Answer from the drawing. Dimensions are ordinates in mm from the lowest x, y and z of the part. A direction names the side the tool comes from. Give positions to 0.01 mm unless a question says otherwise; leave off trailing zeros. Order: outer loops, then holes, each group sorted by start corner. A loop starts at its lowest first (then second) coordinate and runs counter-clockwise, first axis right, second up. Notation, with made-up numbers: (50.25, -28) - (60.25, -28) arc R23 cw to (60.25, -20) - close; hole circle Ø2 at (55, -27.5). An arc over 180 degrees is marked (long way). Answer in a Markdown table with one row per item. Add a question column.
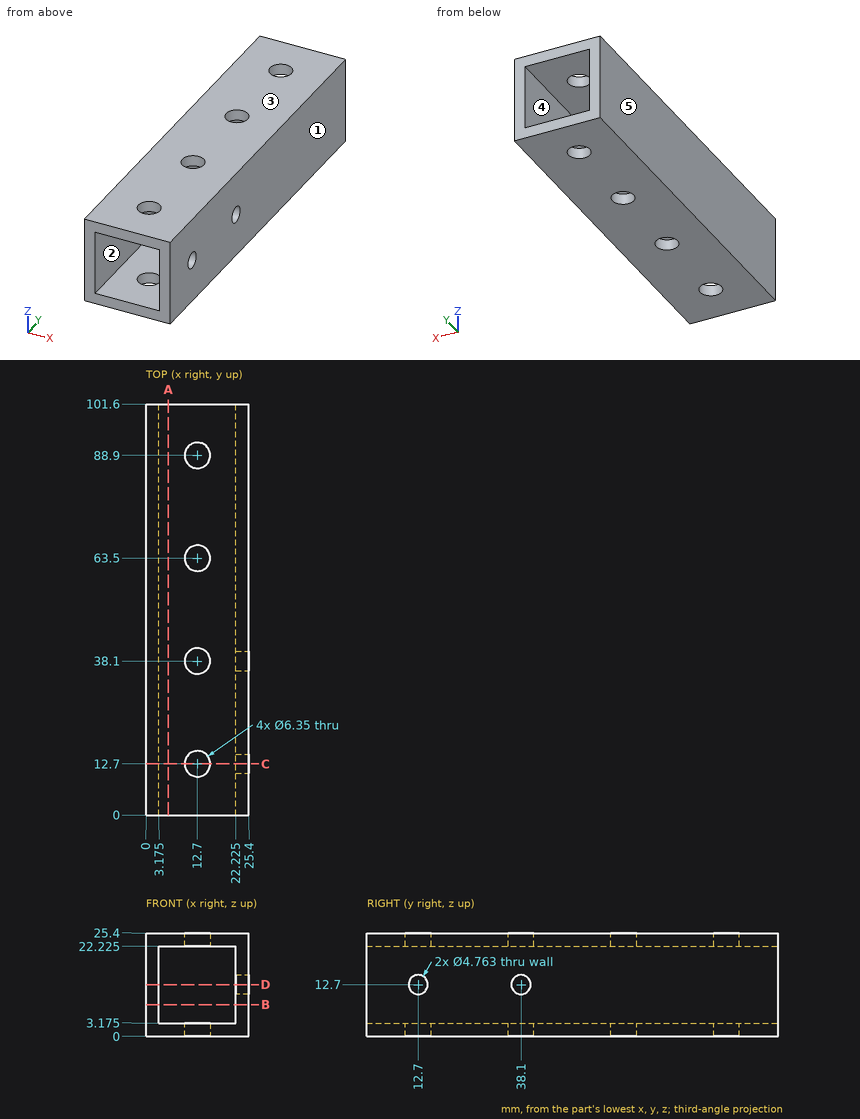
(1) Each of these flat-tipped pins is pushed along its axis until it touches: P1, Ø2, axis at x = 14.5, y = 36.5, coming from the -Z side; P2, Ø4, axis at y = 12.7, z = 12.7, coming from the +X side (1 decimal). Where does it stop, or does it pass through?
(2) Find section C-C, the plane y = 12.7. Write down the section's boundary in (x, z) (1 decimal), plus the area to 3 significant figures.
(3) Find section A-A, the plane x = 5.5. Write down the section's boundary in (y, z) (1 decimal).
(4) Find section B-B, the plane z = 7.75. Write down the section's boundary in (x, y) (1 decimal).
(5) Straight lines are drawn through the part: line 1 (Y direction, x = 12.7, z = 23.2) (1 decimal); line 2 (X direction, y = 37, z = 20.25) (1 decimal). For each, find the intervals that lie inside material, in ascending order.
(6) The mould has two halves that part along X. Classify the marked faces 1, 2 and 3: +X half, -X half, draft (parallel to the pull), parting line (faces both ways), or undercut.
(7) Find section D-D, the plane z = 12.7. Write down the section's boundary in (x, y) (1 decimal).
(8) For the marked faces 4 and 5, determine the directions among +Z, -Z, +X, -X, +Y, -Y from which every point of the face is accessible in a straight line to the end or side of a thin tool.
Answer key:
| question | item | result |
|---|---|---|
| 1 | P1 | z = 0 |
| 1 | P2 | x = 3.2 |
| 2 | outline | (0, 0) - (9.5, 0) - (9.5, 3.2) - (3.2, 3.2) - (3.2, 22.2) - (9.5, 22.2) - (9.5, 25.4) - (0, 25.4) - close; (15.9, 0) - (25.4, 0) - (25.4, 10.3) - (22.2, 10.3) - (22.2, 3.2) - (15.9, 3.2) - close; (15.9, 22.2) - (22.2, 22.2) - (22.2, 15.1) - (25.4, 15.1) - (25.4, 25.4) - (15.9, 25.4) - close |
| 2 | area | 227 mm² |
| 3 | outline | (0, 0) - (101.6, 0) - (101.6, 3.2) - (0, 3.2) - close; (0, 22.2) - (101.6, 22.2) - (101.6, 25.4) - (0, 25.4) - close |
| 4 | outline | (0, 0) - (3.2, 0) - (3.2, 101.6) - (0, 101.6) - close; (22.2, 0) - (25.4, 0) - (25.4, 101.6) - (22.2, 101.6) - close |
| 5 | line 1 | 0 to 9.5, 15.9 to 34.9, 41.3 to 60.3, 66.7 to 85.7, 92.1 to 101.6 |
| 5 | line 2 | 0 to 3.2, 22.2 to 25.4 |
| 6 | face 1 | +X half |
| 6 | face 2 | undercut |
| 6 | face 3 | draft |
| 7 | outline | (0, 0) - (3.2, 0) - (3.2, 101.6) - (0, 101.6) - close; (22.2, 0) - (25.4, 0) - (25.4, 10.3) - (22.2, 10.3) - close; (22.2, 15.1) - (25.4, 15.1) - (25.4, 35.7) - (22.2, 35.7) - close; (22.2, 40.5) - (25.4, 40.5) - (25.4, 101.6) - (22.2, 101.6) - close |
| 8 | face 4 | +Y, -Y |
| 8 | face 5 | +Z, -Z, -X, +Y, -Y |
